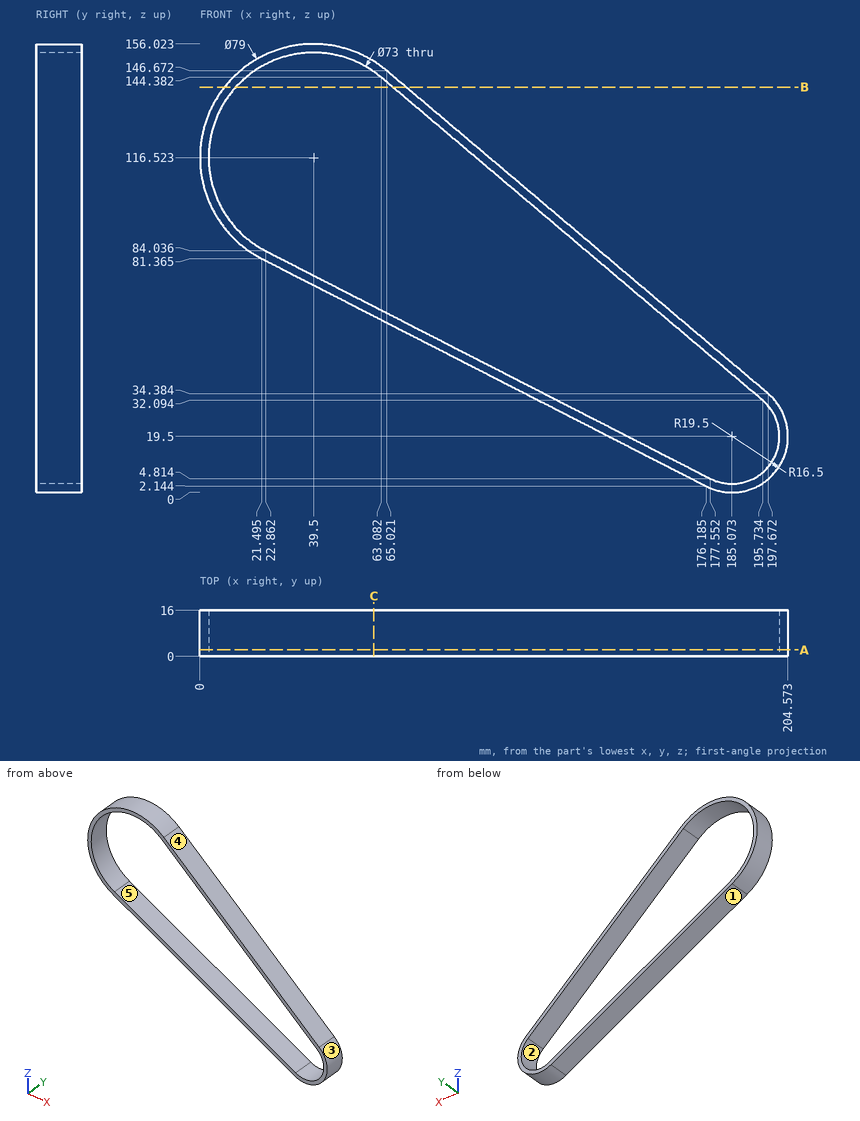
For this review, use the dimensioned drawing (mm, ordinates from the lowest corner) and the shaded views. A direction names the side the tool comes from. Round coordinates to 2 decimals unless told otherwise and drop trailing zeros. Write each loop counter-clockwise with the first axis right and the second up, starting at its lowest first coordinate (ties: lowest second). Pieces come first, ordered by that corner, then holes. Notation, with made-up numbers: (-40, 59.5) -> (4, 59.5) arc R22 ccw to (4, 81.5) -> close; hole circle Ø4 at (62, -32). An arc over 180 degrees is marked (long way). Answer in a Markdown table with one row per item.
Q1. Clearance check with flat-ended pins moving along their axes: pin 1 Ø6 at (x, y) = (109.5, 12) entering from -Z; pin 2 Ø1 at (x, y) = (99, 6) entering from -Z; pin 3 Ø4 at (y, z) = (12, 27.5) entering from -X. State where each tip first meets the part, or that it passes through.
The answers:
| item | result |
|---|---|
| pin 1 | z = 34.76 |
| pin 2 | z = 41.42 |
| pin 3 | x = 122.77 |
Q2. To check wall thickness, follow L1, parallel to Z at x = 112, y = 7 (1 decimal); L2, parallel to Z at x = 86, y = 2 (1 decimal); L3, parallel to X at y = 1.75, z = 41 (1 decimal). State the ranges of each line that lie inside material, in increasing order. Write a range as [from, to].
The answers:
| item | result |
|---|---|
| L1 | [35, 38.4], [103, 106.9] |
| L2 | [48.3, 51.7], [125, 128.9] |
| L3 | [100.3, 106.9], [185.2, 189.9] |
Q3. For the marked faces 4 and 5, list the 3-axis set-ups (+Z, -Z, +X, -X, +Y, -Y) from which the entire face can be reached by the end or side of a thin tool; tool diameter is ignored.
The answers:
| item | result |
|---|---|
| face 4 | +Z, +X, +Y, -Y |
| face 5 | +Y, -Y |
Q4. Take a section at C-C, the plane x = 60.5. State the section outline as (y, z) points.
The answers:
| item | result |
|---|---|
| outline | (0, 61.39) -> (16, 61.39) -> (16, 64.76) -> (0, 64.76) -> close; (0, 146.38) -> (16, 146.38) -> (16, 149.98) -> (0, 149.98) -> close |
Q5. Take a section at B-B, the plane z = 141. State the section outline as (x, y) points.
The answers:
| item | result |
|---|---|
| outline | (8.5, 0) -> (12.42, 0) -> (12.42, 16) -> (8.5, 16) -> close; (67.08, 0) -> (71.72, 0) -> (71.72, 16) -> (67.08, 16) -> close |
Q6. Draft analysis for pull direction Z (two halves, no side actions). For the marked faces 1, 2 and 3, state which applies: +Z half, -Z half, draft (parallel to the pull), parting line (faces both ways), or undercut.
The answers:
| item | result |
|---|---|
| face 1 | -Z half |
| face 2 | undercut |
| face 3 | parting line |
Q7. Take a section at A-A, the plane y = 2.25. State the section outline as (x, z) points (1 decimal).
The answers:
| item | result |
|---|---|
| outline | (21.5, 81.4) -> (176.2, 2.1) arc R19.5 ccw to (197.7, 34.4) -> (65, 146.7) arc R39.5 ccw (long way) to start; hole (22.9, 84) -> (177.6, 4.8) arc R16.5 ccw to (195.7, 32.1) -> (63.1, 144.4) arc R36.5 ccw (long way) to start |
